Work out the finished part from the listing and answer in its coordinate system (mm). A direction names the side the tool comes from. Round coordinates to 2 decimals unless told otherwise and drop trailing zeros. Loops run counter-clockwise (first coordinate to the right, second up) from the corner with the lowest first, then second, coordinate; pieces in that order, holes last. Notation, with made-up numbers: (52, 84.25) -> (86, 84.25) arc R28 cw to (86, 106.25) -> close; hole circle Ø9 at (54, -29.75). An arc over 180 degrees is marked (long way). Use one line per item in the form item = value.
```python
from build123d import *

# Parameters (mm, degrees)
SKETCH1_W                = 155
SKETCH1_H                = 80
BOSS_EXTRUDE1_DEPTH      = 5
SKETCH2_W                = 71.2978
SKETCH2_H                = 27.1018
SCREEN_CUTOUT_DEPTH      = 6
SKETCH2_3_R              = 1.5
SKETCH2_3_W              = 71.2978
SKETCH2_3_H              = 27.1018
CUT_EXTRUDE4_DEPTH       = 2.9
SKETCH3_R                = 8.1
ULTRASOUND_CUTOUTS_DEPTH = 6
SKETCH3_3_R              = 8.1
SKETCH3_3_R_2            = 1.190625
CUT_EXTRUDE2_DEPTH       = 3.175
SKETCH5_W                = 12
SKETCH5_H                = 5
US_CLOCK_CUTOUT_DEPTH    = 4
SKETCH6_W                = 10
SKETCH6_H                = 3.5
US_PIN_CUTOUT_DEPTH      = 2
SKETCH9_R                = 3.15
MAGNET_HOLES_DEPTH       = 2.1
FILLET1_R                = 6
SKETCH10_W               = 46.5
SKETCH10_H               = 57
KEYPAD_CUTOUT_DEPTH      = 6
SKETCH11_W               = 46.5
SKETCH11_H               = 57
SKETCH11_W_2             = 52
SKETCH11_H_2             = 64
SKETCH11_W_3             = 38
SKETCH11_H_3             = 6
CUT_EXTRUDE1_DEPTH       = 1.5
FILLET3_R                = 2
FILLET4_R                = 2
SKETCH12_R               = 1.5
CUT_EXTRUDE3_DEPTH       = 2.9


with BuildPart() as part:
    # Sketch1 → Boss-Extrude1 (new body)
    with BuildSketch(Plane(origin=(0, 0, 0), x_dir=(1, 0, 0), z_dir=(0, 1, 0))):
        Rectangle(SKETCH1_W, SKETCH1_H)
    extrude(amount=BOSS_EXTRUDE1_DEPTH)

    # Sketch2 → Screen Cutout (cut, through all)
    with BuildSketch(Plane(origin=(0, 0, 0), x_dir=(1, 0, 0), z_dir=(0, 1, 0))):
        with Locations((-27.2029, 15.22)):
            Rectangle(SKETCH2_W, SKETCH2_H)
    extrude(amount=SCREEN_CUTOUT_DEPTH, mode=Mode.SUBTRACT)

    # Sketch2_3 → Cut-Extrude4 (cut)
    with BuildSketch(Plane(origin=(0, 0, 0), x_dir=(1, 0, 0), z_dir=(0, 1, 0))):
        with Locations((-64.96, -0.02)):
            Circle(SKETCH2_3_R)
        with Locations((9.97, -0.02)):
            Circle(SKETCH2_3_R)
        with Locations((9.97, 30.46)):
            Circle(SKETCH2_3_R)
        with Locations((-64.96, 30.46)):
            Circle(SKETCH2_3_R)
        with Locations((-27.2029, 15.22)):
            Rectangle(SKETCH2_3_W, SKETCH2_3_H)
    extrude(amount=CUT_EXTRUDE4_DEPTH, mode=Mode.SUBTRACT)

    # Sketch3 → Ultrasound Cutouts (cut, through all)
    with BuildSketch(Plane(origin=(0, 0, 0), x_dir=(1, 0, 0), z_dir=(0, 1, 0))):
        with Locations((-40.2029, -20)):
            Circle(SKETCH3_R)
        with Locations((-14.2029, -20)):
            Circle(SKETCH3_R)
    extrude(amount=ULTRASOUND_CUTOUTS_DEPTH, mode=Mode.SUBTRACT)

    # Sketch3_3 → Cut-Extrude2 (cut)
    with BuildSketch(Plane(origin=(0, 0, 0), x_dir=(1, 0, 0), z_dir=(0, 1, 0))):
        with Locations((-40.2029, -20)):
            Circle(SKETCH3_3_R)
        with Locations((-14.2029, -20)):
            Circle(SKETCH3_3_R)
        with Locations((-48.3529, -11.45)):
            Circle(SKETCH3_3_R_2)
        with Locations((-6.0529, -11.45)):
            Circle(SKETCH3_3_R_2)
        with Locations((-6.0529, -28.55)):
            Circle(SKETCH3_3_R_2)
        with Locations((-48.3529, -28.55)):
            Circle(SKETCH3_3_R_2)
    extrude(amount=CUT_EXTRUDE2_DEPTH, mode=Mode.SUBTRACT)

    # Sketch5 → US Clock cutout (cut)
    with BuildSketch(Plane.XZ):
        with Locations((-27.471992442, 27.55)):
            Rectangle(SKETCH5_W, SKETCH5_H)
    extrude(amount=-US_CLOCK_CUTOUT_DEPTH, mode=Mode.SUBTRACT)

    # Sketch6 → US Pin cutout (cut)
    with BuildSketch(Plane.XZ):
        with Locations((-27.471992442, 11.55)):
            Rectangle(SKETCH6_W, SKETCH6_H)
    extrude(amount=-US_PIN_CUTOUT_DEPTH, mode=Mode.SUBTRACT)

    # Sketch9 → Magnet Holes (cut)
    with BuildSketch(Plane(origin=(0, 0.2, 0), x_dir=(-1, 0, 0), z_dir=(0, -1, 0))):
        with Locations((-71.5, 34)):
            Circle(SKETCH9_R)
        with Locations((71.5, 34)):
            Circle(SKETCH9_R)
        with Locations((-71.5, -34)):
            Circle(SKETCH9_R)
        with Locations((71.5, -34)):
            Circle(SKETCH9_R)
    extrude(amount=-MAGNET_HOLES_DEPTH, mode=Mode.SUBTRACT)

    # Fillet1
    fillet1_edges = [part.edges().sort_by_distance(p)[0] for p in [
        (77.5, 2.5, 40),
        (-77.5, 2.5, 40),
        (-77.5, 2.5, -40),
        (77.5, 2.5, -40),
    ]]
    fillet(fillet1_edges, radius=FILLET1_R)

    # Sketch10 → Keypad cutout (cut, through all)
    with BuildSketch(Plane(origin=(0, 5, 0), x_dir=(1, 0, 0), z_dir=(0, 1, 0))):
        with Locations((39.696, 3.5)):
            Rectangle(SKETCH10_W, SKETCH10_H)
    extrude(amount=-KEYPAD_CUTOUT_DEPTH, mode=Mode.SUBTRACT)

    # Sketch11 → Cut-Extrude1 (cut)
    with BuildSketch(Plane.XZ):
        with Locations((39.696, -3.5)):
            Rectangle(SKETCH11_W, SKETCH11_H)
        with Locations((39.696, -3.5)):
            Rectangle(SKETCH11_W_2, SKETCH11_H_2)
        with Locations((39.696, -3.5)):
            Rectangle(SKETCH11_W, SKETCH11_H, mode=Mode.SUBTRACT)
        with Locations((39.696, 31.5)):
            Rectangle(SKETCH11_W_3, SKETCH11_H_3)
    extrude(amount=-CUT_EXTRUDE1_DEPTH, mode=Mode.SUBTRACT)

    # Fillet3
    fillet3_edges = [part.edges().sort_by_distance(p)[0] for p in [
        (13.696, 0.75, -35.5),
        (13.696, 0.75, 28.5),
        (65.696, 0.75, 28.5),
        (65.696, 0.75, -35.5),
    ]]
    fillet(fillet3_edges, radius=FILLET3_R)

    # Fillet4
    fillet4_edges = [part.edges().sort_by_distance(p)[0] for p in [
        (16.446, 3.25, -32),
        (62.946, 3.25, -32),
        (16.446, 3.25, 25),
        (62.946, 3.25, 25),
    ]]
    fillet(fillet4_edges, radius=FILLET4_R)

    # Sketch12 → Cut-Extrude3 (cut)
    with BuildSketch(Plane.XZ.offset(-1.5)):
        with Locations((63.092012723, -34.123666466)):
            Circle(SKETCH12_R)
        with Locations((15.839087894, -34.123666466)):
            Circle(SKETCH12_R)
        with Locations((15.839087894, 26.403006737)):
            Circle(SKETCH12_R)
        with Locations((63.092012723, 26.403006737)):
            Circle(SKETCH12_R)
    extrude(amount=-CUT_EXTRUDE3_DEPTH, mode=Mode.SUBTRACT)


solid = part.part
```
(1) Find section C-C, the plane x = 9.97. Write down the section's boundary in (y, z).
Completed:
outline = (0, -40) -> (5, -40) -> (5, 40) -> (0, 40) -> (0, 1.52) -> (2.9, 1.52) -> (2.9, -1.48) -> (0, -1.48) -> (0, -28.96) -> (2.9, -28.96) -> (2.9, -31.96) -> (0, -31.96) -> close
(2) Consider L1, parallel to X at y = 4, z = -4; L2, parallel to Z at x = -71.5, y = 1.75; L3, parallel to X at y = 0.8, z = 34. Determine where each line is inside the solid, lowest interval first.
Completed:
L1 = -77.5 to -62.85, 8.45 to 16.45, 62.95 to 77.5
L2 = -40 to -37.15, -30.85 to 30.85, 37.15 to 40
L3 = -77.5 to -74.65, -68.35 to 20.7, 58.7 to 68.35, 74.65 to 77.5
(3) Find section A-A, the plane x = 47. Write down the section's boundary in (y, z).
Completed:
outline = (0, -40) -> (5, -40) -> (5, -32) -> (1.5, -32) -> (1.5, -35.5) -> (0, -35.5) -> close; (0, 34.5) -> (1.5, 34.5) -> (1.5, 25) -> (5, 25) -> (5, 40) -> (0, 40) -> close
(4) Given P1, Ø0.7, axis at x = -6.5, z = 28.5, coming from the -Y side (3 decimals); P2, Ø2, axis at x = -45.5, z = 22.5, coming from the +Y side; P3, Ø0.9, axis at x = 10.5, z = 0.5, coming from the -Y side; P4, Ø1.5, axis at x = -29.5, z = 27.5, coming from the -Y side, each flat-ended and moving along its own axis, determine where each tip first touches the part or whether it passes through.
Completed:
P1 = 3.175
P2 = through
P3 = 2.9
P4 = 4
(5) Find section B-B, the plane z = -13.5. Write down the section's boundary in (x, y), then the cut area to 3 significant figures.
Completed:
outline = (-77.5, 0) -> (-62.85, 0) -> (-62.85, 5) -> (-77.5, 5) -> close; (8.45, 0) -> (13.7, 0) -> (13.7, 1.5) -> (16.45, 1.5) -> (16.45, 5) -> (8.45, 5) -> close; (62.95, 1.5) -> (65.7, 1.5) -> (65.7, 0) -> (77.5, 0) -> (77.5, 5) -> (62.95, 5) -> close
area = 178 mm2
(6) For a pull along Y with two mould halves and no side action, classify faces 6 (the cylindrical face through (74.647, 1.235, -34.138)), 7 (the flat face through (-28, 2, 12)), 8 (the flat face through (77.5, 2, 0)) as +Y half, -Y half, draft (parallel to the pull), parting line (faces both ways), or undercut.
Completed:
face_6 = undercut
face_7 = -Y half
face_8 = draft
(7) For faces 1 (the cylindrical face through (75.696, 2.535, 38.289)), 2 (the flat face through (8.446, 2, -15)), 3 (the cylindrical face through (10.66, 1.43, -29.13)), 4 (the cylindrical face through (75.696, 2.535, -38.289)), 5 (the flat face through (72, 0.2, 34)), determine the directions among +Z, -Z, +X, -X, +Y, -Y from which every point of the face is accessible in a straight line to the end or side of a thin tool.
Completed:
face_1 = +Z, +X, +Y, -Y
face_2 = +Y, -Y
face_3 = -Y
face_4 = -Z, +X, +Y, -Y
face_5 = none
